Verification items for this drawing (mm, ordinates from the low corner). Coordinates: 2 decimals unless noted, no trailing zeros. Write each loop counter-clockwise with the first axis right and the second up, starting at its lowest first coordinate (ties: lowest second). Pieces come first, ordered by that corner, then holes. Notation, with made-up numbers: M -16,47.25 L 18,47.25 A34 cw 18,84.25 Z; hole C -10.5,52.5 d5. An arc over 180 degrees is marked long. Write each question's results on one line, items separated by ' | '.
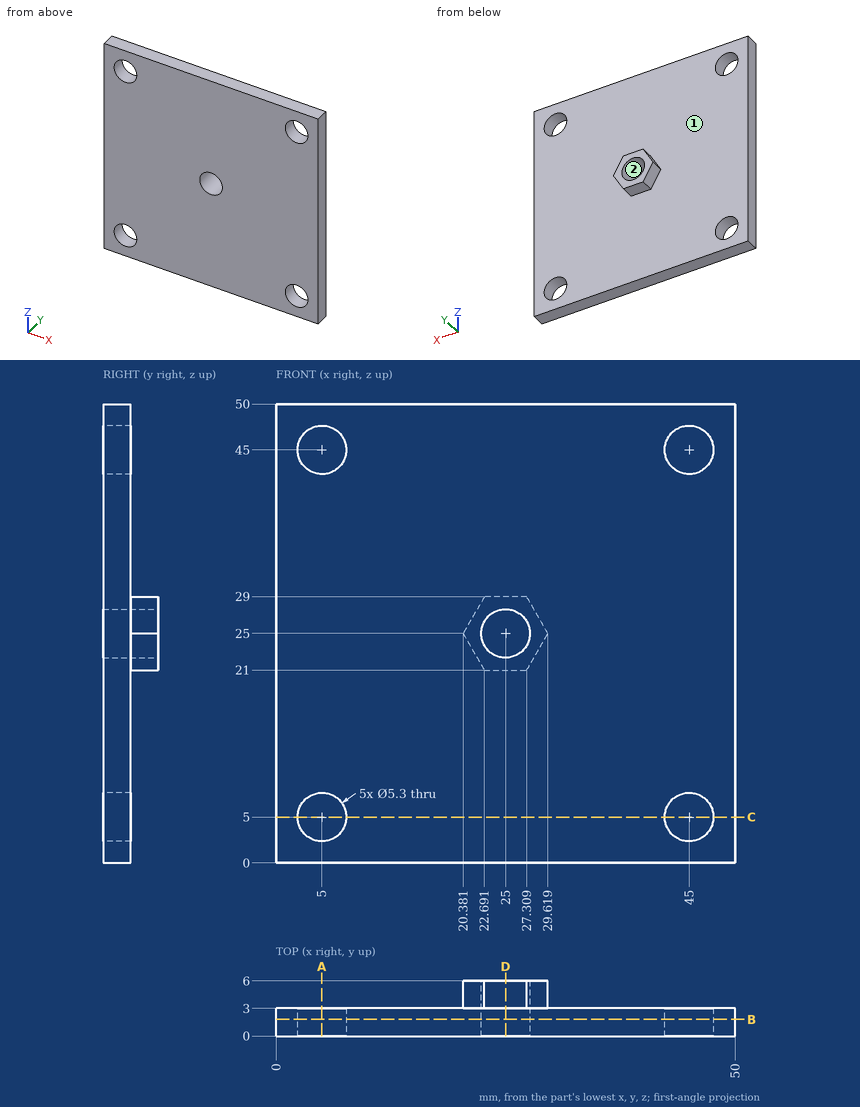
Q1. Scan lines: probe 1 along Z at (x, y) = (5, 1.4); probe 2 along Z at (x, y) = (25, 1.3); probe 3 along Y at (x, z) = (44, 30.5). Record each from-to range of solid material in increasing order.
Geometry check:
probe 1: z = 0 to 2.35, 7.65 to 42.35, 47.65 to 50 | probe 2: z = 0 to 22.35, 27.65 to 50 | probe 3: y = 0 to 3
Q2. Mould release check, pull along Z, two halves, no side actions. Record for the marked faces 1 and 2: pulls with the +Z half, pulls with the -Z half, needs draft (parallel to the pull), parting line crosses it, or undercut.
Geometry check:
face 1: needs draft | face 2: undercut
Q3. Sectioned sample at B-B on y = 1.8. Record the cut outline in (x, z), and give its area (3 significant figures).
Geometry check:
outline: M 0,0 L 50,0 L 50,50 L 0,50 Z; hole C 5,5 d5.3; hole C 5,45 d5.3; hole C 25,25 d5.3; hole C 45,5 d5.3; hole C 45,45 d5.3 | area: 2,390 mm2
Q4. Sectioned sample at D-D on x = 25. Record the cut outline in (y, z).
Geometry check:
outline: M 0,0 L 3,0 L 3,21 L 6,21 L 6,22.35 L 0,22.35 Z; M 0,27.65 L 6,27.65 L 6,29 L 3,29 L 3,50 L 0,50 Z
Q5. Depth check by flat-ended pin: P1, Ø1.5, axis at x = 25.5, y = 4.5, coming from the +Z side; P2, Ø1, axis at x = 38, z = 30, coming from the +Y side; P3, Ø2.5, axis at x = 24.5, y = 5, coming from the -Z side; P4, Ø7, axis at x = 25, z = 25, coming from the -Y side. Enter the tip coordinate at first touch or a pass-through.
Geometry check:
P1: stops at z = 29 | P2: stops at y = 3 | P3: stops at z = 21 | P4: stops at y = 0
Q6. Sectioned sample at A-A on x = 5. Record the cut outline in (y, z), and give its area (3 significant figures).
Geometry check:
outline: M 0,0 L 3,0 L 3,2.35 L 0,2.35 Z; M 0,7.65 L 3,7.65 L 3,42.35 L 0,42.35 Z; M 0,47.65 L 3,47.65 L 3,50 L 0,50 Z | area: 118 mm2
Q7. Sectioned sample at C-C on z = 5. Record the cut outline in (x, y), and give its area (3 significant figures).
Geometry check:
outline: M 0,0 L 2.35,0 L 2.35,3 L 0,3 Z; M 7.65,0 L 42.35,0 L 42.35,3 L 7.65,3 Z; M 47.65,0 L 50,0 L 50,3 L 47.65,3 Z | area: 118 mm2
